```python
from build123d import *

# Parameters (mm, degrees)
SKETCH1_W           = 70
SKETCH1_H           = 20
SKETCH1_R           = 2
SKETCH1_R_2         = 1.5
SKETCH1_W_2         = 3
SKETCH1_H_2         = 10
BOSS_EXTRUDE1_DEPTH = 3


with BuildPart() as part:
    # Sketch1 → Boss-Extrude1 (new body)
    with BuildSketch(Plane(origin=(0, 0, 0), x_dir=(1, 0, 0), z_dir=(0, 1, 0))):
        with Locations((35, 10)):
            Rectangle(SKETCH1_W, SKETCH1_H)
        with Locations(Location((10, 10, 0), (0, 0, 270))):
            Circle(SKETCH1_R, mode=Mode.SUBTRACT)
        with Locations(Location((27.5, 10, 0), (0, 0, 270))):
            Circle(SKETCH1_R_2, mode=Mode.SUBTRACT)
        with Locations(Location((60, 10, 0), (0, 0, 90))):
            Circle(SKETCH1_R, mode=Mode.SUBTRACT)
        with Locations(Location((42.5, 10, 0), (0, 0, 90))):
            Circle(SKETCH1_R_2, mode=Mode.SUBTRACT)
        with Locations((20, 10)):
            Rectangle(SKETCH1_W_2, SKETCH1_H_2, mode=Mode.SUBTRACT)
        with Locations((50, 10)):
            Rectangle(SKETCH1_W_2, SKETCH1_H_2, mode=Mode.SUBTRACT)
    extrude(amount=BOSS_EXTRUDE1_DEPTH)


solid = part.part
```
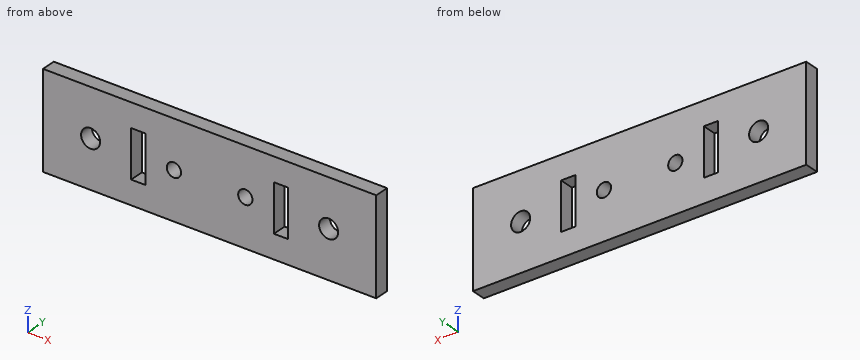
Design review of the part built by this model. Coordinates are the model's own, in mm. Coordinates: 2 decimals unless noted, no trailing zeros. Loops run counter-clockwise (first coordinate to the right, second up) from the corner with the lowest first, then second, coordinate; pieces in that order, holes last. Notation, with made-up numbers: M 16.25,-22 L 39.25,-22 A7 cw 39.25,-13 Z; hole C -29,34 d7. An arc over 180 degrees is marked long. One line per question, with ' | ' between items.
(1) We need section C-C (y = 1.65). Give the boundary of the cut face in (x, z).
Filled in:
outline: M 0,-20 L 70,-20 L 70,0 L 0,0 Z; hole C 10,-10 d4; hole M 18.5,-15 L 21.5,-15 L 21.5,-5 L 18.5,-5 Z; hole C 27.5,-10 d3; hole C 42.5,-10 d3; hole M 48.5,-15 L 51.5,-15 L 51.5,-5 L 48.5,-5 Z; hole C 60,-10 d4
(2) For pin 1 Ø1.8 at (x, z) = (42.5, -10) entering from -Y, flat-tipped, find the tip position at first contact; note if it passes through.
Filled in:
pin 1: passes through
(3) We need section A-A (x = 42.5). Give the boundary of the cut face in (y, z), and give its area (3 significant figures).
Filled in:
outline: M 0,-20 L 3,-20 L 3,-11.5 L 0,-11.5 Z; M 0,-8.5 L 3,-8.5 L 3,0 L 0,0 Z | area: 51.0 mm^2
(4) Wall thickness on probe 1 along X at (y, z) = (1.6, -13); probe 2 along Z at (x, y) = (60, 1.25); probe 3 along Z at (x, y) = (50, 1.35): over which ranges is each line inside the solid? List them lowest first.
Filled in:
probe 1: x = 0 to 18.5, 21.5 to 48.5, 51.5 to 70 | probe 2: z = -20 to -12, -8 to 0 | probe 3: z = -20 to -15, -5 to 0
(5) We need section D-D (x = 10). Give the boundary of the cut face in (y, z).
Filled in:
outline: M 0,-20 L 3,-20 L 3,-12 L 0,-12 Z; M 0,-8 L 3,-8 L 3,0 L 0,0 Z
(6) We need section B-B (z = -10). Give the boundary of the cut face in (x, y), and give its area (3 significant figures).
Filled in:
outline: M 0,0 L 8,0 L 8,3 L 0,3 Z; M 12,0 L 18.5,0 L 18.5,3 L 12,3 Z; M 21.5,0 L 26,0 L 26,3 L 21.5,3 Z; M 29,0 L 41,0 L 41,3 L 29,3 Z; M 44,0 L 48.5,0 L 48.5,3 L 44,3 Z; M 51.5,0 L 58,0 L 58,3 L 51.5,3 Z; M 62,0 L 70,0 L 70,3 L 62,3 Z | area: 150 mm^2
